Autodesk Inventor part; units mm, degrees
ref_plane "YZ Plane" through (0, 0, 0) normal (1, 0, 0) x (0, 1, 0)
ref_plane "XZ Plane" through (0, 0, 0) normal (0, 1, 0) x (-1, 0, 0)
ref_plane "XY Plane" through (0, 0, 0) normal (0, 0, 1) x (1, 0, 0)
sketch "Sketch1" plane through (0, 0, 0) normal (0, 0, 1) x (1, 0, 0)
  line L0 (-188.0565, 0) -> (188.0565, 0)
  line L1 (-188.0565, 0) -> (-188.0565, 8)
  line L2 (-188.0565, 8) -> (183.0565, 8)
  line L3 (183.0565, 8) -> (183.0565, 15)
  line L4 (183.0565, 15) -> (188.0565, 15)
  line L5 (188.0565, 15) -> (188.0565, 0)
  circle A0 centre (-183.0565, 0) radius 1.75
  point P0 (0, 0)
  point P1 (0, 0)
  point P2 (183.0565, 8.25)
  dimension "d0" = 376.113
  dimension "d1" = 16
  dimension "d2" = 5
  dimension "d3" = 30
  dimension "d8" = 3.5
  dimension "d9" = 5
  dimension "d12" = 0.25
revolve "Revolution1" add sketch "Sketch1" angle 360 about axis through (-188.0565, 0, 0) along (1, 0, 0) picked at (-182.9862, 0.5791) contours A0 L0 L1 L2 L3 L4 L5 | L0 A0
fillet "Fillet1" radius 1 1 edges at (-188.0565, -8, 0)
chamfer "Chamfer1" distance 1 angle 45 3 edges at (188.0565, -15, 0) (-187.0565, -8, 0) (-188.0565, -7, 0)
extrude "Extrusion2" cut sketch "Sketch1" against normal through all both and the other way through all contours A0 L0 | L0 A0
properties part number "PWTR-0158" material "Stainless Steel"
Verification items for the finished model (mm, model axes). A direction names the side the tool comes from. Coordinates: 2 decimals unless noted, no trailing zeros. Order: outer loops, then holes, each group sorted by start corner. A loop starts at its lowest first (then second) coordinate and runs counter-clockwise, first axis right, second up. Notation, with made-up numbers: M 79,35 L 88,35 A20 cw 88,73 Z; hole C 86,84 d10. An arc over 180 degrees is marked long. One line per item, written item: value. Start each with the question number.
Item 1: Access from +Z, -Z, +X, -X, +Y, -Y to the whole of each face (thin tool, end or side, straight path). Record for faces 1 (the flat face through (-188.056, 0, 0)), 2 (the flat face through (183.056, 6, -6)).
Item 2: Thickness scan on probe 1 along X at (y, z) = (0, 0.5); probe 2 along X at (y, z) = (9.75, 10); probe 3 along Y at (x, z) = (-119, -1). Record the ranges inside material, lowest first.
Item 3: Sectioned sample at B-B on x = -21.5. Record the cut outline in (y, z).
Item 4: Depth check by flat-ended pin: P1, Ø4, axis at y = -10.5, z = -2, coming from the -X side; P2, Ø1.5, axis at x = -56.5, y = 7.5, coming from the -Z side; P3, Ø3, axis at x = -183.06, y = 0, coming from the -Z side; P4, Ø6, axis at x = 137.5, y = -10, coming from the -Z side. Enter the tip coordinate at first touch or a pass-through.
Item 5: Sectioned sample at A-A on z = 0. Record the cut outline in (x, y), then the cut area to 3 significant figures.
Calculated:
1. face 1: +Z, -Z, -X, +Y, -Y
1. face 2: -X
2. probe 1: -188.06 to -184.81, -181.31 to 188.06
2. probe 2: 183.06 to 188.06
2. probe 3: -7.94 to 7.94
3. outline: C 0,0 d16
4. P1: x = 183.06
4. P2: z = -4.29
4. P3: through
4. P4: z = -3.87
5. outline: M -188.06,-7 A1 ccw -187.06,-8 L 183.06,-8 L 183.06,-15 L 187.06,-15 L 188.06,-14 L 188.06,14 L 187.06,15 L 183.06,15 L 183.06,8 L -187.06,8 A1 ccw -188.06,7 Z; hole C -183.06,0 d3.5
5. area: 6,080 mm^2
